The listing builds one solid part. Answer for the finished solid, in the listing's coordinates (mm). A direction names the side the tool comes from. Round coordinates to 2 decimals unless told otherwise and drop trailing zeros. Write each loop counter-clockwise with the first axis right and the second up, starting at its lowest first coordinate (ties: lowest second). Pieces come first, ordered by that corner, then holes.
(1) Find the intervals of material crossed by probe 1 along Z at (x, y) = (21.5, 0); probe 2 along Y at (x, z) = (22.5, -2.75); probe 3 along Z at (x, y) = (21, -31), in increasing order.
(2) For faces 1 (the face through (14.544, 3.284, 1.445)), 2 (the face through (15, -24, 1)), determine the directions among +Z, -Z, +X, -X, +Y, -Y from which every point of the face is accessible in a straight line to the end or side of a thin tool.
(3) A cutting plane is placed at C-C, the plane y = -38. Give the vertices of the cut face in (x, z).
(4) A cutting plane is placed at A-A, the plane y = 0. Give the vertices of the cut face in (x, z).
(5) A cutting plane is placed at B-B, the plane x = 12.75. Give the vertices of the cut face in (y, z).
(6) The mould has two halves that part along Z. Classify faces 3 (the face through (14.54, -0.02, -3.73)), 4 (the face through (14.5, -41, -0.5)), 5 (the face through (14.5, -2, -2.5)): +Z half, -Z half, draft (parallel to the pull), parting line (faces both ways), or undercut.
(7) Each of these flat-tipped pins is pushed along its axis until it touches: pin 1 Ø15 at (x, y) = (19, -18.5) entering from +Z; pin 2 Ø0.5 at (x, z) = (11, 3) entering from -Y; pin 3 Ø0.5 at (x, z) = (11.5, -2.5) entering from +Y; pin 4 Ø1.6 at (y, z) = (0, 0) entering from +X. Where does it stop, or does it pass through?
from build123d import *

# Parameters (mm, degrees)
SKETCH_R  = 1
PAD_DEPTH = 29.5


with BuildPart() as part:
    # Sketch → Pad (new body)
    with BuildSketch(Plane.YZ):
        with BuildLine():
            ThreePointArc((-39.994398, 0.999984), (-40.705123, 0.709085), (-41, 0))
            Line((-41, 0), (-41, -1))
            ThreePointArc((-41, -1), (-40.707107, -1.707107), (-40, -2))
            Line((-40, -2), (-2, -2))
            Line((-2, -2), (-2, -3))
            ThreePointArc((-2, -3), (-1.91611, -3.791945), (-1.213507, -4.166863))
            ThreePointArc((-1.213507, -4.166863), (0, -3.728848), (1.213507, -4.166863))
            ThreePointArc((1.213507, -4.166863), (1.818438, -3.726112), (2, -3))
            Line((2, -3), (2, -2))
            Line((2, -2), (2.654702, -2))
            ThreePointArc((2.654702, -2), (3.614511, -0.992973), (3.171248, 0.325684))
            Line((3.171248, 0.325684), (3.4, 2.595785))
            Line((3.4, 2.595785), (4.4, 2.595785))
            Line((4.4, 2.595785), (4.4, 3.74))
            ThreePointArc((4.4, 3.74), (4.312132, 3.952132), (4.1, 4.04))
            Line((4.1, 4.04), (-7, 4.04))
            ThreePointArc((-7, 4.04), (-7.58987, 3.847498), (-7.952638, 3.344107))
            Line((-7.952638, 3.344107), (-7.952638, 2.298428))
            ThreePointArc((-7.952638, 2.298428), (-8.36641, 1.418293), (-9.244398, 0.999984))
            Line((-9.244398, 0.999984), (-39.994398, 0.999984))
        make_face()
        Circle(SKETCH_R, mode=Mode.SUBTRACT)
    extrude(amount=PAD_DEPTH)


solid = part.part
Solutions:
1. probe 1: z = -3.73 to -1, 1 to 4.04
1. probe 2: y = -2 to 2
1. probe 3: z = -2 to 1
2. face 1: +X, -X, +Y
2. face 2: +Z, +X, -X, -Y
3. outline: (0, -2) - (29.5, -2) - (29.5, 1) - (0, 1) - close
4. outline: (0, -3.73) - (29.5, -3.73) - (29.5, -1) - (0, -1) - close; (0, 1) - (29.5, 1) - (29.5, 4.04) - (0, 4.04) - close
5. outline: (-41, -1) arc R1 ccw to (-40, -2) - (-2, -2) - (-2, -3) arc R0.85 ccw to (-1.21, -4.17) arc R1.9 cw to (1.21, -4.17) arc R1.1 ccw to (2, -3) - (2, -2) - (2.65, -2) arc R1.35 ccw to (3.17, 0.33) - (3.4, 2.6) - (4.4, 2.6) - (4.4, 3.74) arc R0.3 ccw to (4.1, 4.04) - (-7, 4.04) arc R1 ccw to (-7.95, 3.34) - (-7.95, 2.3) arc R1.44 cw to (-9.24, 1) - (-39.99, 1) arc R1 ccw to (-41, 0) - close; hole circle Ø2 at (0, 0)
6. face 3: -Z half
6. face 4: draft
6. face 5: undercut
7. pin 1: stops at z = 1
7. pin 2: stops at y = -7.95
7. pin 3: stops at y = 2
7. pin 4: passes through
